The listing builds one solid part. Answer for the finished solid, in the listing's coordinates (mm). A direction names the side the tool comes from. Coordinates: 2 decimals unless noted, no trailing zeros. Order: outer loops, then holes, each group sorted by start corner. A loop starts at its lowest first (then second) coordinate and runs counter-clockwise, first axis right, second up. Notation, with made-up numbers: (27, 37.25) -> (42, 37.25) arc R17 ccw to (42, 70.25) -> close; hole circle Ø4 at (39.25, -33). An arc over 180 degrees is marked (long way). Write each question's results on one line, items separated by ' | '. Start each with the question number.
(1) The part is cut by section D-D, the plane x = -9. Give the vertices of the cut face in (y, z), then the cut area to 3 significant figures.
(2) A tool of negligible diameter and unlimited length cuts with its end or side. For faces 4 (the face through (15, 42, 2)), 5 (the face through (-14.26, 9.483, 2.028)), 6 (the face through (-15, 42, 2)), from which of +Z, -Z, +X, -X, +Y, -Y can it reach the whole face along a straight path? Write none if from no direction.
(3) Straight lines are drawn through the part: L1, parallel to Y at x = -9, z = 1.7; L2, parallel to Y at x = 14, z = 2.8; L3, parallel to X at y = 8, z = 2. For each, find the intervals that lie inside material, in ascending order.
(4) Given pin 1 (3 mm diameter, centred on x = -14, y = 7.5, fed in from +Z); pin 2 (2 mm diameter, centred on y = 35, z = 1.5, fed in from -X); pin 3 (2 mm diameter, centred on y = 22, z = 1.5, fed in from -X), each flat-ended and moving along its own axis, determine where each tip first touches the part or whether it passes through.
(5) The part is cut by section C-C, the plane x = -14. Give the vertices of the cut face in (y, z), then the cut area to 3 significant figures.
(6) The part is cut by section A-A, the plane z = 1.1. Count the separate pieces of the cut face and the enclosed holes in it, then the cut area to 3 significant figures.
(7) Determine the mould class of faces 1 (the face through (0, 23, 0)), 2 (the face through (-9.325, 51.536, 2.028)), 3 (the face through (0, 59, 2)) for opening direction Y: +Y half, -Y half, draft (parallel to the pull), parting line (faces both ways), or undercut.
(8) The part is cut by section B-B, the plane y = 7.5. Give the vertices of the cut face in (x, z).
```python
from build123d import *

# Parameters (mm, degrees)
EXTRUDE_1_DEPTH     = 4
SKETCH_2_R          = 1.5
CUT_EXTRUDE_1_DEPTH = 65.202803677
SKETCH_3_R          = 2
CUT_EXTRUDE_2_DEPTH = 65.202803677
FILLET_1_R          = 10


with BuildPart() as part:
    # 草图1 → 凸台-拉伸1 (new body)
    with BuildSketch(Plane.XY):
        Polygon((25, 0), (-25, 0), (-25, 15), (-15, 15), (-15, 59), (15, 59), (15, 15), (25, 15), align=None)
    extrude(amount=EXTRUDE_1_DEPTH)

    # 草图2 → 切除-拉伸1 (cut, through all)
    with BuildSketch(Plane.XY.offset(4)):
        with Locations((-9, 53)):
            Circle(SKETCH_2_R)
        with Locations((-9, 35)):
            Circle(SKETCH_2_R)
        with Locations((9, 35)):
            Circle(SKETCH_2_R)
        with Locations((9, 53)):
            Circle(SKETCH_2_R)
    extrude(amount=-CUT_EXTRUDE_1_DEPTH, mode=Mode.SUBTRACT)

    # 草图3 → 切除-拉伸2 (cut, through all)
    with BuildSketch(Plane.XY.offset(4)):
        with Locations((-14, 7.5)):
            Circle(SKETCH_3_R)
        with Locations(Location((14, 7.5, 0), (0, 0, 180))):
            Circle(SKETCH_3_R)
    extrude(amount=-CUT_EXTRUDE_2_DEPTH, mode=Mode.SUBTRACT)

    # 圆角1
    fillet_1_edges = [part.edges().sort_by_distance(p)[0] for p in [
        (-15, 15, 2),
        (15, 15, 2),
    ]]
    fillet(fillet_1_edges, radius=FILLET_1_R - 0.0001)  # a hair under: the kernel refuses the full size


solid = part.part
```
Established:
1) outline: (0, 0) -> (33.5, 0) -> (33.5, 4) -> (0, 4) -> close; (36.5, 0) -> (51.5, 0) -> (51.5, 4) -> (36.5, 4) -> close; (54.5, 0) -> (59, 0) -> (59, 4) -> (54.5, 4) -> close | area: 212 mm^2
2) face 4: +Z, -Z, +X, +Y | face 5: +Z, -Z | face 6: +Z, -Z, -X, +Y
3) L1: y = 0 to 33.5, 36.5 to 51.5, 54.5 to 59 | L2: y = 0 to 5.5, 9.5 to 59 | L3: x = -25 to -15.94, -12.06 to 12.06, 15.94 to 25
4) pin 1: passes through | pin 2: stops at x = -15 | pin 3: stops at x = -15.83
5) outline: (0, 0) -> (5.5, 0) -> (5.5, 4) -> (0, 4) -> close; (9.5, 0) -> (59, 0) -> (59, 4) -> (9.5, 4) -> close | area: 220 mm^2
6) separate pieces: 1 | enclosed holes: 6 | area: 2,060 mm^2
7) face 1: draft | face 2: undercut | face 3: +Y half
8) outline: (-25, 0) -> (-16, 0) -> (-16, 4) -> (-25, 4) -> close; (-12, 0) -> (12, 0) -> (12, 4) -> (-12, 4) -> close; (16, 0) -> (25, 0) -> (25, 4) -> (16, 4) -> close
